Autodesk Inventor part; units mm, degrees
ref_plane "作業平面1" through (-9.5, -10, 1000) normal (0, 0, 1) x (1, 0, 0)
ref_plane "YZ Plane" through (0, 0, 0) normal (1, 0, 0) x (0, 1, 0)
ref_plane "XZ Plane" through (0, 0, 0) normal (0, 1, 0) x (-1, 0, 0)
ref_plane "作業平面1" through (-9.5, -10, 1000) normal (0, 0, 1) x (1, 0, 0)
sketch "スケッチ1" plane through (-9.5, -10, 1000) normal (0, 0, 1) x (1, 0, 0)
  line L0 (7.35, 18.5) -> (7.35, 20)
  line L1 (7.35, 20) -> (0, 20)
  arc A0 (0, 20) -> (-0.5, 19.5) centre (0, 19.5) ccw
  line L2 (-0.5, 19.5) -> (-0.5, 12.15)
  line L3 (-0.5, 12.15) -> (1, 12.15)
  line L4 (1, 12.15) -> (1, 14.15)
  line L5 (1, 14.15) -> (4.7, 14.15)
  line L6 (4.7, 14.15) -> (4.7, 12.15)
  line L7 (4.7, 12.15) -> (6.5, 12.15)
  line L8 (6.5, 12.15) -> (6.5, 7.85)
  line L9 (6.5, 7.85) -> (4.7, 7.85)
  line L10 (4.7, 7.85) -> (4.7, 5.85)
  line L11 (4.7, 5.85) -> (1, 5.85)
  line L12 (1, 5.85) -> (1, 7.85)
  line L13 (1, 7.85) -> (-0.5, 7.85)
  line L14 (-0.5, 7.85) -> (-0.5, 0.5)
  arc A1 (-0.5, 0.5) -> (0, 0) centre (0, 0.5) ccw
  line L15 (0, 0) -> (19, 0)
  arc A2 (19, 0) -> (19.5, 0.5) centre (19, 0.5) ccw
  line L16 (19.5, 0.5) -> (19.5, 7.85)
  line L17 (19.5, 7.85) -> (18, 7.85)
  line L18 (18, 7.85) -> (18, 5.85)
  line L19 (18, 5.85) -> (14.3, 5.85)
  line L20 (14.3, 5.85) -> (14.3, 7.85)
  line L21 (14.3, 7.85) -> (12.5, 7.85)
  line L22 (12.5, 7.85) -> (12.5, 12.15)
  line L23 (12.5, 12.15) -> (14.3, 12.15)
  line L24 (14.3, 12.15) -> (14.3, 14.15)
  line L25 (14.3, 14.15) -> (18, 14.15)
  line L26 (18, 14.15) -> (18, 12.15)
  line L27 (18, 12.15) -> (19.5, 12.15)
  line L28 (19.5, 12.15) -> (19.5, 19.5)
  arc A3 (19.5, 19.5) -> (19, 20) centre (19, 19.5) ccw
  line L29 (19, 20) -> (11.65, 20)
  line L30 (11.65, 20) -> (11.65, 18.5)
  line L31 (11.65, 18.5) -> (13.65, 18.5)
  line L32 (13.65, 18.5) -> (13.65, 14.8)
  line L33 (13.65, 14.8) -> (11.65, 14.8)
  line L34 (11.65, 14.8) -> (11.65, 13)
  line L35 (11.65, 13) -> (7.35, 13)
  line L36 (7.35, 13) -> (7.35, 14.8)
  line L37 (7.35, 14.8) -> (5.35, 14.8)
  line L38 (5.35, 14.8) -> (5.35, 18.5)
  line L39 (5.35, 18.5) -> (7.35, 18.5)
  arc A4 (11.6496, 6.4) -> (11.0496, 7) centre (11.0496, 6.4) ccw
  line L40 (11.6496, 6.4) -> (11.6496, 5.5)
  arc A5 (11.6496, 5.5) -> (11.9496, 5.2) centre (11.9496, 5.5) ccw
  line L41 (11.9496, 5.2) -> (13.3496, 5.2)
  arc A6 (13.6496, 4.9) -> (13.3496, 5.2) centre (13.3496, 4.9) ccw
  arc A7 (13.6496, 4.9) -> (13.7891, 4.5617) centre (13.9391, 4.8215) ccw
  line L42 (13.7891, 4.5617) -> (14.3769, 4.2223)
  arc A8 (14.3769, 4.2223) -> (15.0013, 4.3244) centre (14.6267, 4.6555) ccw
  arc A9 (15.0029, 1.6738) -> (15.0013, 4.3244) centre (16.5, 3) ccw
  arc A10 (15.0029, 1.6738) -> (14.3787, 1.7753) centre (14.6287, 1.3422) ccw
  line L43 (14.3787, 1.7753) -> (13.9715, 1.5402)
  arc A11 (13.8215, 1.5) -> (13.9715, 1.5402) centre (13.8215, 1.8) ccw
  line L44 (13.8215, 1.5) -> (5.1785, 1.5)
  arc A12 (5.0285, 1.5402) -> (5.1785, 1.5) centre (5.1785, 1.8) ccw
  line L45 (5.0285, 1.5402) -> (4.6213, 1.7753)
  arc A13 (4.6213, 1.7753) -> (3.9971, 1.6738) centre (4.3713, 1.3422) ccw
  arc A14 (3.9971, 4.3262) -> (3.9971, 1.6738) centre (2.5, 3) ccw
  arc A15 (3.9971, 4.3262) -> (4.6213, 4.2247) centre (4.3713, 4.6578) ccw
  line L46 (4.6213, 4.2247) -> (5.2, 4.5588)
  arc A16 (5.2, 4.5588) -> (5.35, 4.8187) centre (5.05, 4.8187) ccw
  arc A17 (5.6395, 5.1972) -> (5.35, 4.8187) centre (5.6395, 4.8972) ccw
  line L47 (5.6395, 5.1972) -> (7.05, 5.1972)
  arc A18 (7.05, 5.1972) -> (7.35, 5.4972) centre (7.05, 5.4972) ccw
  line L48 (7.35, 5.4972) -> (7.35, 6.4)
  arc A19 (7.95, 7) -> (7.35, 6.4) centre (7.95, 6.4) ccw
  line L49 (7.95, 7) -> (11.0496, 7)
  circle A20 centre (2.5, 17) radius 2
  circle A21 centre (16.5, 17) radius 2
  circle A22 centre (9.5, 10) radius 1.65
  point P0 (9.5, 10)
extrude "押し出し1" add sketch "スケッチ1" along normal blind 40
properties part number "AFSF-2020-4"
Geometry check sheet. Reference: the model listing, model coordinates, mm. A direction names the side the tool comes from. Give positions to 0.01 mm unless a question says otherwise; leave off trailing zeros. Order: outer loops, then holes, each group sorted by start corner. A loop starts at its lowest first (then second) coordinate and runs counter-clockwise, first axis right, second up. Notation, with made-up numbers: (-21, 38) - (18, 38) arc R27 cw to (18, 61) - close; hole circle Ø5 at (-0.5, 40.25). An arc over 180 degrees is marked (long way). Write item = value, one per line. Start each with the question number.
1) Section check C-C (x = 7). Enter the section's corners in (y, z), then the cut area to 3 significant figures.
2) Access from +Z, -Z, +X, -X, +Y, -Y to the whole of each face (thin tool, end or side, straight path). Record for faces 4 (the flat face through (9, 2.15, 1020)), 5 (the flat face through (-4, 2.15, 1020)), 6 (the flat face through (-7, -4.15, 1020)).
3) Section check A-A (y = -7). Enter the section's corners in (x, z), then the cut area to 3 significant figures.
4) Draft check along Y on faces 1 (the flat face through (2.15, 9, 1020)), 2 (the flat face through (-6, 10, 1020)), 3 (the flat face through (7, -4.15, 1020)). Enter one of: released by +Y, released by -Y, zero draft, split by the parting line, or undercut.
5) Section check B-B (x = 0). Enter the section's corners in (y, z).
6) Scan lines: L1, parallel to Y at x = -3.25, z = 1012; L2, parallel to Y at x = -7, z = 1027.5. Record each from-to range of solid material in increasing order.
Geometry check:
q1.outline = (-10, 1000) - (-9, 1000) - (-9, 1040) - (-10, 1040) - close; (-5, 1000) - (-4.15, 1000) - (-4.15, 1040) - (-5, 1040) - close; (4.15, 1000) - (5, 1000) - (5, 1040) - (4.15, 1040) - close; (9, 1000) - (10, 1000) - (10, 1040) - (9, 1040) - close
q1.area = 148 mm2
q2.face_4 = +Z, -Z, +X
q2.face_5 = +Z, -Z, -X
q2.face_6 = +Z, -Z
q3.outline = (-10, 1000) - (-9, 1000) - (-9, 1040) - (-10, 1040) - close; (9, 1000) - (10, 1000) - (10, 1040) - (9, 1040) - close
q3.area = 80.0 mm2
q4.face_1 = zero draft
q4.face_2 = released by +Y
q4.face_3 = undercut
q5.outline = (-10, 1000) - (-8.5, 1000) - (-8.5, 1040) - (-10, 1040) - close; (-3, 1000) - (-1.65, 1000) - (-1.65, 1040) - (-3, 1040) - close; (1.65, 1000) - (3, 1000) - (3, 1040) - (1.65, 1040) - close
q6.L1 = -10 to -8.5, -4.8 to -2.15, 2.15 to 4.8, 8.5 to 10
q6.L2 = -10 to -9, -5 to -4.15, 4.15 to 5, 9 to 10
